```python
from build123d import *

# Parameters (mm, degrees)
F0_W     = 50
F0_H     = 50
F1_DEPTH = 25
F4_DEPTH = 50
F7_DEPTH = 50


with BuildPart() as f1:
    # F0 (on Front) → F1 (new body, symmetric)
    with BuildSketch(Plane.XZ):
        Rectangle(F0_W, F0_H)
    extrude(amount=F1_DEPTH, both=True)

    # F3 (on offset) → F4 (cut)
    with BuildSketch(Plane.XZ.offset(25)):
        Polygon((-8, 25), (-25, 25), (-25, -25), align=None)
        Polygon((4.149, 0), (0, 15), (-4.149486, 0), (0, 0), align=None)
        Polygon((8, 25), (25, -25), (25, 25), align=None)
        Polygon((-5.240043, -5.117772), (-12, -25), (12, -25), (5.240043, -5.117772), align=None)
    extrude(amount=-F4_DEPTH, mode=Mode.SUBTRACT)

    # F6 (on offset) → F7 (cut)
    with BuildSketch(Plane.XY.offset(25)):
        with BuildLine():
            Line((25, 25), (6.959901, 25))
            ThreePointArc((6.959901, 25), (19.459901, 12.5), (6.959901, 0))
            Line((6.959901, 0), (7.5, 0))
            Line((7.5, 0), (12.5, 0))
            ThreePointArc((12.5, 0), (21.338835, -3.661165), (25, -12.5))
            Line((25, -12.5), (25, 25))
        make_face()
        with BuildLine():
            ThreePointArc((25, -12.5), (21.338835, -21.338835), (12.5, -25))
            Line((12.5, -25), (25, -25))
            Line((25, -25), (25, -12.5))
        make_face()
        with BuildLine():
            Line((7.486049, -3), (-17.513951, -3))
            Line((-17.513951, -3), (-17.513951, -22))
            Line((-17.513951, -22), (7.486049, -22))
            ThreePointArc((7.486049, -22), (16.986049, -12.5), (7.486049, -3))
        make_face()
        with BuildLine():
            Line((2.459141, 21.999886), (-17.540099, 21.999886))
            Line((-17.540099, 21.999886), (-17.540099, 2.999886))
            Line((-17.540099, 2.999886), (2.459141, 3.174202))
            ThreePointArc((2.459141, 3.174202), (11.871983, 12.587044), (2.459141, 21.999886))
        make_face()
    extrude(amount=-F7_DEPTH, mode=Mode.SUBTRACT)


solid = f1.part
```
Build history of the part. All positions in model axes, mm. A direction names the side the tool comes from. Round coordinates to 2 decimals unless told otherwise and drop trailing zeros. Write each loop counter-clockwise with the first axis right and the second up, starting at its lowest first coordinate (ties: lowest second). Pieces come first, ordered by that corner, then holes.
1) Drill centre lines: probe 1 along Y at (x, z) = (2, 8.5); probe 2 along Y at (x, z) = (-7, -2); probe 3 along Z at (x, y) = (4.5, 22). Where is each one in solid material? Low to high.
2) 3-axis set-ups, long thin cutter, end or side, ignore diameter. For faces 5 (the flat face through (-17.54, 13, -14)), 6 (the flat face through (0, 23, -5.118)), 7 (the flat face through (-2.046, -23.521, 7.605)): which of +Z, -Z, +X, -X, +Y, -Y reach the whole face in a straight line?
3) Band-saw the part on C-C, the plane z = -16. List the corners of the cut face in (x, y).
4) Band-saw the part on D-D, the plane x = -10. List the corners of the cut face in (y, z), and give its area (3 significant figures).
5) Band-saw the part on B-B, the plane x = 1. List the corners of the cut face in (y, z).
6) Band-saw the part on A-A, the plane y = 17. List the corners of the cut face in (x, z), and give its area (3 significant figures).
7) Mould opens along X. For faces 1 (the cylindrical face through (17.658, -1.114, -14.53)), 2 (the cylindrical face through (11.87, 12.38, 0.54)), 3 (the flat face through (-9, 25, 0)), 4 (the flat face through (-5, -3, 6)) say: +X half, -X half, draft (parallel to the pull), parting line (faces both ways), or undercut.
8) Pin check, flat tips, straight feed: pin 1 (3.5 mm diameter, centred on x = -0.5, y = -0.5, fed in from -Z); pin 2 (1.5 mm diameter, centred on x = 19, z = -14.5, fed in from +Y); pin 3 (4 mm diameter, centred on x = 5, z = -16, fed in from +Y); pin 4 (3 mm diameter, centred on x = 9, z = -3, fed in from +Y). Stop position of each tip, or through.
Ans:
1. probe 1: y = -25 to -22, -3 to 3.17, 22 to 25
1. probe 2: y = -25 to -22, -3 to 3.09, 22 to 25
1. probe 3: z = -5.12 to 25
2. face 5: +Z, -Z
2. face 6: -Z, +Y, -Y
2. face 7: +Y, -Y
3. outline: (-21.94, -25) - (-8.94, -25) - (-8.94, -22) - (-17.51, -22) - (-17.51, -3) - (-8.94, -3) - (-8.94, 3.07) - (-17.54, 3) - (-17.54, 22) - (-8.94, 22) - (-8.94, 25) - (-21.94, 25) - close; (8.94, -25) - (12.5, -25) arc R12.5 ccw to (21.94, -20.69) - (21.94, -4.31) arc R12.5 ccw to (12.5, 0) - (8.94, 0) - (8.94, -3.11) arc R9.5 cw to (8.94, -21.89) - close; (8.94, 0.16) arc R12.5 ccw to (8.94, 24.84) - (8.94, 19.41) arc R9.41 cw to (8.94, 5.76) - close
4. outline: (-25, -19.12) - (-22, -19.12) - (-22, 19.12) - (-25, 19.12) - close; (-3, -19.12) - (3.07, -19.12) - (3.07, 19.12) - (-3, 19.12) - close; (22, -19.12) - (25, -19.12) - (25, 19.12) - (22, 19.12) - close
4. area: 461 mm2
5. outline: (-25, -5.12) - (-22, -5.12) - (-22, 0) - (-25, 0) - close; (-25, 11.38) - (-22, 11.38) - (-22, 25) - (-25, 25) - close; (-3, -5.12) - (3.16, -5.12) - (3.16, 0) - (-3, 0) - close; (-3, 11.38) - (3.16, 11.38) - (3.16, 25) - (-3, 25) - close; (22, -5.12) - (25, -5.12) - (25, 0) - (22, 0) - close; (22, 11.38) - (25, 11.38) - (25, 25) - (22, 25) - close
6. outline: (-25, -25) - (-17.54, -25) - (-17.54, -3.06) - close; (10.77, -21.39) - (12, -25) - (18.62, -25) - (18.62, -6.24) - (10.77, 16.84) - close
6. area: 317 mm2
7. face 1: +X half
7. face 2: undercut
7. face 3: draft
7. face 4: undercut
8. pin 1: stops at z = -5.12
8. pin 2: stops at y = 17.87
8. pin 3: passes through
8. pin 4: stops at y = 24.99
